from build123d import *

# Parameters (mm, degrees)
ESQUISSE1_R             = 31.75
ESQUISSE1_R_2           = 12.7
ESQUISSE1_R_3           = 2.25
BOSS_EXTRU_1_DEPTH      = 19.05
BOSS_EXTRU_2_DEPTH      = 19.05
ESQUISSE3_R             = 3.175
ENL_V_MAT_EXTRU_1_DEPTH = 90.603345812
ESQUISSE4_R             = 3.175
ENL_V_MAT_EXTRU_2_DEPTH = 90.603345812
ESQUISSE5_R             = 3.175
ENL_V_MAT_EXTRU_3_DEPTH = 70.418897208
CONG_1_R                = 1


with BuildPart() as part:
    # Esquisse1 → Boss.-Extru.1 (new body)
    with BuildSketch(Plane.XY):
        Circle(ESQUISSE1_R)
        Circle(ESQUISSE1_R_2, mode=Mode.SUBTRACT)
        with Locations((0, 25.4)):
            Circle(ESQUISSE1_R_3, mode=Mode.SUBTRACT)
        with Locations((-21.997045256, -12.7)):
            Circle(ESQUISSE1_R_3, mode=Mode.SUBTRACT)
        with Locations((21.997045256, -12.7)):
            Circle(ESQUISSE1_R_3, mode=Mode.SUBTRACT)
    extrude(amount=BOSS_EXTRU_1_DEPTH)

    # Esquisse2 → Boss.-Extru.2 (add)
    with BuildSketch(Plane.XY.offset(19.05)):
        Polygon((42.868897208, 35.748891971), (21.467304731, 23.392676794), (17.187758818, 26.6953825), (40.368897208, 40.07901899), align=None)
        Polygon((30.992304731, 6.894892851), (31.712758818, 1.53734452), (54.893897208, 14.92098101), (52.393897208, 19.251108029), align=None)
        Polygon((14.525, -55), (14.525, -28.23272702), (9.525, -30.287569645), (9.525, -55), align=None)
        Polygon((-9.525, -30.287569645), (-14.525, -28.23272702), (-14.525, -55), (-9.525, -55), align=None)
        Polygon((-54.893897208, 14.92098101), (-31.712758818, 1.53734452), (-30.992304731, 6.894892851), (-52.393897208, 19.251108029), align=None)
        Polygon((-21.467304731, 23.392676794), (-17.187758818, 26.6953825), (-40.368897208, 40.07901899), (-42.868897208, 35.748891971), align=None)
    extrude(amount=-BOSS_EXTRU_2_DEPTH)

    # Esquisse3 → Enlèv. mat.-Extru.1 (cut, through all)
    with BuildSketch(Plane(origin=(7.2625, 12.57901899, 0), x_dir=(0.866025404, -0.5, 0), z_dir=(0.5, 0.866025404, 0))):
        with Locations((-47.0625, -6.35)):
            Circle(ESQUISSE3_R)
    extrude(amount=-ENL_V_MAT_EXTRU_1_DEPTH, mode=Mode.SUBTRACT)

    # Esquisse4 → Enlèv. mat.-Extru.2 (cut, through all)
    with BuildSketch(Plane(origin=(-7.2625, 12.57901899, 0), x_dir=(0.866025404, 0.5, 0), z_dir=(-0.5, 0.866025404, 0))):
        with Locations((47.0625, -6.35)):
            Circle(ESQUISSE4_R)
    extrude(amount=-ENL_V_MAT_EXTRU_2_DEPTH, mode=Mode.SUBTRACT)

    # Esquisse5 → Enlèv. mat.-Extru.3 (cut, through all)
    with BuildSketch(Plane(origin=(14.525, 0, 0), x_dir=(0, 0, -1), z_dir=(1, 0, 0))):
        with Locations((-6.35, -47.0625)):
            Circle(ESQUISSE5_R)
    extrude(amount=-ENL_V_MAT_EXTRU_3_DEPTH, mode=Mode.SUBTRACT)

    # Congé1
    cong_1_edges = [part.edges().sort_by_distance(p)[0] for p in [
        (40.368897208, 40.07901899, 9.525),
        (42.868897208, 35.748891971, 9.525),
        (21.467304731, 23.392676794, 9.525),
        (17.187758818, 26.6953825, 9.525),
        (30.992304731, 6.894892851, 9.525),
        (52.393897208, 19.251108029, 9.525),
        (54.893897208, 14.92098101, 9.525),
        (31.712758818, 1.53734452, 9.525),
        (14.525, -55, 9.525),
        (9.525, -55, 9.525),
        (9.525, -30.287569645, 9.525),
        (14.525, -28.23272702, 9.525),
        (-9.525, -30.287569645, 9.525),
        (-9.525, -55, 9.525),
        (-14.525, -55, 9.525),
        (-14.525, -28.23272702, 9.525),
        (-54.893897208, 14.92098101, 9.525),
        (-52.393897208, 19.251108029, 9.525),
        (-30.992304731, 6.894892851, 9.525),
        (-31.712758818, 1.53734452, 9.525),
        (-21.467304731, 23.392676794, 9.525),
        (-42.868897208, 35.748891971, 9.525),
        (-40.368897208, 40.07901899, 9.525),
        (-17.187758818, 26.6953825, 9.525),
    ]]
    fillet(cong_1_edges, radius=CONG_1_R)


solid = part.part
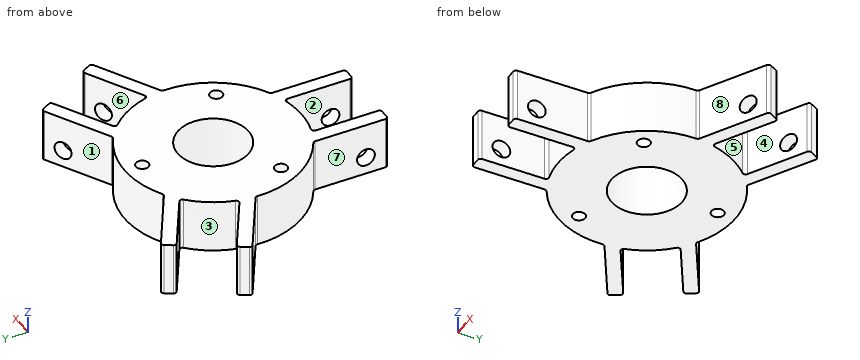
Verification items for the finished model (mm, model axes). Face numbers are marked on the shaded views. A direction names the side the tool comes from. Coordinates: 2 decimals unless noted, no trailing zeros. Loops run counter-clockwise (first coordinate to the right, second up) from the corner with the lowest first, then second, coordinate; pieces in that order, holes last. Notation, with made-up numbers: (35, -4) -> (61, -4) arc R21 cw to (61, 11) -> close; hole circle Ø5 at (76, 33). An arc over 180 degrees is marked (long way). Answer as a JSON object with one key per item and string values. Group by question number.
Item 1: Tool access check on the marked faces 1, 2, 3 and 4. Record the directions out of +Z, -Z, +X, -X, +Y, -Y that give a thin tool (end or side, any length) a straight path to the whole face; none if there is none.
Item 2: Mould release check, pull along Y, two halves, no side actions. Record for the marked faces 5, 6, 7 and 8: +Y half, -Y half, draft (parallel to the pull), parting line (faces both ways), or undercut.
Item 3: Sectioned sample at A-A on y = -36. Record the boundary of the cut face in (x, z) (3 decimals).
Item 4: Depth check by flat-ended pin: pin 1 (8 mm diameter, centred on x = 17.5, z = 10, fed in from +Y); pin 2 (5.5 mm diameter, centred on y = -36, z = 5.5, fed in from -X) (3 decimals); pin 3 (3 mm diameter, centred on y = -28.5, z = 10.5, fed in from -X). Enter the tip coordinate at first touch or a pass-through.
Item 5: Sectioned sample at C-C on z = 6.35. State how many separate pieces and enclosed holes the cut face has, plus the area to 3 significant figures.
Item 6: Scan lines: probe 1 along Y at (x, z) = (0, 4); probe 2 along X at (y, z) = (-13.5, 11); probe 3 along X at (y, z) = (-34.5, 16.75) (3 decimals). Record each from-to range of solid material in increasing order.
Item 7: Sectioned sample at B-B on x = 5. Record the boundary of the cut face in (y, z), plus the area to 3 significant figures.
Evaluation:
{
 "1": {"face 1": "+Z, -Z, +Y", "face 2": "+Z, -Z, -Y", "face 3": "+Z, -Z", "face 4": "+Z, -Z, +X"},
 "2": {"face 5": "undercut", "face 6": "undercut", "face 7": "draft", "face 8": "-Y half"},
 "3": {"outline": "(-14.525, 0) -> (-9.525, 0) -> (-9.525, 19.05) -> (-14.525, 19.05) -> close; (9.525, 0) -> (14.525, 0) -> (14.525, 19.05) -> (9.525, 19.05) -> close"},
 "4": {"pin 1": "stops at y = 29.19", "pin 2": "stops at x = -14.525", "pin 3": "stops at x = -16.71"},
 "5": {"separate pieces": "7", "enclosed holes": "4", "area": "3,190 mm²"},
 "6": {"probe 1": "y = -31.75 to -12.7, 12.7 to 23.15, 27.65 to 31.75", "probe 2": "x = -28.74 to -24.1, -19.89 to 19.89, 24.1 to 28.74", "probe 3": "x = -14.525 to -9.525, 9.525 to 14.525"},
 "7": {"outline": "(-31.35, 0) -> (-11.67, 0) -> (-11.67, 19.05) -> (-31.35, 19.05) -> close; (11.67, 0) -> (31.35, 0) -> (31.35, 19.05) -> (11.67, 19.05) -> close", "area": "750 mm²"}
}
